Read the model definition and answer for the solid it produces. Units are mm, in the model's axes. A direction names the side the tool comes from. Coordinates: 2 decimals unless noted, no trailing zeros. Write each loop counter-clockwise with the first axis right and the second up, starting at its lowest first coordinate (ties: lowest second). Pieces come first, ordered by that corner, then holes.
1) Determine the mould class of faces 1 (the face through (4, 23, 257.5)), 2 (the face through (4, 5, 4)), 3 (the face through (4, 0, 4)) for opening direction Z: +Z half, -Z half, draft (parallel to the pull), parting line (faces both ways), or undercut.
2) Find the intervals of material crossed by line 1 (Z direction, x = 110.5, y = 29); line 2 (Y direction, x = 18, z = 87.5), in increasing order.
3) This flat-tipped pin is pushed along its axis until it touches: pin 1 Ø5 at (x, z) = (-41, -104.5) entering from -Y. Where does it stop, or does it pass through?
4) The part is cut by section A-A (y = 33). Determine the outline of the cut face in (x, z).
5) The part is cut by section C-C (z = -9). Determine the outline of the cut face in (x, y).
6) The part is cut by section B-B (x = 42). Determine the outline of the cut face in (y, z), then the cut area to 3 significant figures.
7) Which of the six approach directions +Z, -Z, +X, -X, +Y, -Y give full straight-line access (tool end or side, diameter ignored) to faces 4 (the face through (-4, 23, -257.5)), 5 (the face through (-4, 25, -252.5))?
Autodesk Inventor part; units mm, degrees
ref_plane "YZ Plane" through (0, 0, 0) normal (1, 0, 0) x (0, 1, 0)
ref_plane "XZ Plane" through (0, 0, 0) normal (0, 1, 0) x (-1, 0, 0)
ref_plane "XY Plane" through (0, 0, 0) normal (0, 0, 1) x (1, 0, 0)
sketch "スケッチ1" plane through (0, 0, 0) normal (0, 1, 0) x (-1, 0, 0)
  line L0 (-290, 257.5) -> (290, 257.5)
  line L1 (290, 257.5) -> (290, -257.5)
  line L2 (290, -257.5) -> (-290, -257.5)
  line L3 (-290, -257.5) -> (-290, 257.5)
  line L4 (-290, 257.5) -> (290, -257.5) construction
  line L5 (290, 257.5) -> (-290, -257.5) construction
  line L6 (285, 257.5) -> (285, -257.5)
  line L7 (290, -252.5) -> (-290, -252.5)
  line L8 (290, 252.5) -> (-290, 252.5)
  point P0 (0, 0)
  dimension "d0" = 580
  dimension "d1" = 515
  dimension "d2" = 5
  dimension "d3" = 5
  dimension "d4" = 5
extrude "押し出し1" add sketch "スケッチ1" along normal blind 45 contours L0 L6 L8 L3 | L0 L1 L8 L6 | L7 L6 L2 L3 | L7 L1 L2 L6
extrude "押し出し2" add sketch "スケッチ1" along normal blind 5 contours L0 L6 L8 L3 | L8 L6 L7 L3 | L7 L6 L2 L3
fillet "フィレット1" radius 2.5 1 edges at (0, 0, -257.5)
fillet "フィレット2" radius 2.5 1 edges at (0, 0, 257.5)
extrude "押し出し3" add sketch "スケッチ1" along normal blind 5 contours L8 L6 L7 L3 | L8 L1 L7 L6
properties part number "controller_table" material "ステンレス鋼"
Reported:
1. face 1: +Z half
1. face 2: undercut
1. face 3: draft
2. line 1: z = -257.5 to -252.5, 252.5 to 257.5
2. line 2: y = 0 to 5
3. pin 1: stops at y = 0
4. outline: (-290, -257.5) - (290, -257.5) - (290, -252.5) - (-290, -252.5) - close; (-290, 252.5) - (290, 252.5) - (290, 257.5) - (-290, 257.5) - close
5. outline: (-290, 0) - (290, 0) - (290, 5) - (-290, 5) - close
6. outline: (0, -255) arc R2.5 ccw to (2.5, -257.5) - (45, -257.5) - (45, -252.5) - (5, -252.5) - (5, 252.5) - (45, 252.5) - (45, 257.5) - (2.5, 257.5) arc R2.5 ccw to (0, 255) - close
6. area: 2,970 mm2
7. face 4: -Z, +X, -X, +Y, -Y
7. face 5: +X, -X, +Y
